```python
from build123d import *

# Parameters (mm, degrees)
SKETCH_W        = 42.5
SKETCH_H        = 70
SKETCH_R        = 11.15
SKETCH_R_2      = 1.65
SKETCH_R_3      = 2.5
PAD003_DEPTH    = 8
POCKET002_DEPTH = 4.15
SKETCH007_W     = 10
SKETCH007_H     = 70
SKETCH007_R     = 1.65
PAD004_DEPTH    = 12
SKETCH008_R     = 8.5
POCKET003_DEPTH = 12
CHAMFER004_SIZE = 3
SKETCH011_R     = 1.65
PAD005_DEPTH    = 12
CHAMFER005_SIZE = 1
SKETCH012_R     = 1.65
POCKET005_DEPTH = 8.001
SKETCH013_R     = 1.65
POCKET006_DEPTH = 20.001
SKETCH014_R     = 4
SKETCH014_R_2   = 2.5
PAD006_DEPTH    = 0.85
CHAMFER006_SIZE = 0.84
SKETCH015_R     = 1.9
POCKET007_DEPTH = 6
SKETCH016_R     = 3.15
POCKET008_DEPTH = 10.001
SKETCH017_W     = 4
SKETCH017_H     = 12.3
POCKET009_DEPTH = 12
CHAMFER007_SIZE = 1
SKETCH018_W     = 17
SKETCH018_H     = 6.956198
SKETCH018_W_2   = 15
SKETCH018_H_2   = 7.10749
SKETCH018_H_3   = 7.8
PAD007_DEPTH    = 1
CHAMFER008_SIZE = 0.99
SKETCH019_R     = 3.25
POCKET010_DEPTH = 7
SKETCH020_R     = 2
POCKET011_DEPTH = 6
CHAMFER009_SIZE = 0.4
POCKET027_DEPTH = 12
FILLET_R        = 1
SKETCH041_R     = 4.5
SKETCH041_R_2   = 2.5
PAD012_DEPTH    = 7
CHAMFER021_SIZE = 0.4


with BuildPart() as part:
    # Sketch → Pad003 (new body)
    with BuildSketch(Plane.XY):
        with Locations((21.25, 35)):
            Rectangle(SKETCH_W, SKETCH_H)
        with Locations((21.25, 48.75)):
            Circle(SKETCH_R, mode=Mode.SUBTRACT)
        with Locations((5.75, 64.25)):
            Circle(SKETCH_R_2, mode=Mode.SUBTRACT)
        with Locations((36.75, 64.25)):
            Circle(SKETCH_R_2, mode=Mode.SUBTRACT)
        with Locations((5.75, 33.25)):
            Circle(SKETCH_R_2, mode=Mode.SUBTRACT)
        with Locations((36.75, 33.25)):
            Circle(SKETCH_R_2, mode=Mode.SUBTRACT)
        with Locations((17.5, 6.74)):
            Circle(SKETCH_R_3, mode=Mode.SUBTRACT)
    extrude(amount=PAD003_DEPTH)

    # Sketch006 (on Face12 of Pad003) → Pocket002 (cut)
    with BuildSketch(Plane.XY.offset(8)):
        Polygon((42.5, 27.65), (23.35, 27.65), (20.35, 24.65), (20.35, 14.35), (23.35, 11.35), (42.5, 11.35), align=None)
    extrude(amount=-POCKET002_DEPTH, mode=Mode.SUBTRACT)

    # Sketch007 (on Face4 of Pocket002) → Pad004 (join)
    with BuildSketch(Plane.XY.offset(8)):
        with Locations((5, 35)):
            Rectangle(SKETCH007_W, SKETCH007_H)
        with Locations((5.75, 64.25)):
            Circle(SKETCH007_R, mode=Mode.SUBTRACT)
        with Locations((5.75, 33.25)):
            Circle(SKETCH007_R, mode=Mode.SUBTRACT)
    extrude(amount=PAD004_DEPTH)

    # Sketch008 (on Face4 of Pad004) → Pocket003 (cut)
    with BuildSketch(Plane.XY.offset(8)):
        with Locations((17.5, 6.74)):
            Circle(SKETCH008_R)
    extrude(amount=POCKET003_DEPTH, mode=Mode.SUBTRACT)

    # Chamfer004
    chamfer004_edges = [part.edges().sort_by_distance(p)[0] for p in [
        (42.5, 70, 4),
        (0, 70, 4),
    ]]
    chamfer(chamfer004_edges, length=CHAMFER004_SIZE)

    # Sketch011 (on Face5 of Chamfer004) → Pad005 (join)
    with BuildSketch(Plane.XY.offset(8)):
        Polygon((42.5, 67), (39.5, 70), (31.5, 70), (31.5, 59), (42.5, 59), align=None)
        with Locations((36.75, 64.25)):
            Circle(SKETCH011_R, mode=Mode.SUBTRACT)
    extrude(amount=PAD005_DEPTH)

    # Chamfer005
    chamfer005_edges = [part.edges().sort_by_distance(p)[0] for p in [
        (42.5, 59, 14),
        (31.5, 59, 14),
        (31.5, 70, 14),
        (10, 70, 14),
        (10, 0, 14),
    ]]
    chamfer(chamfer005_edges, length=CHAMFER005_SIZE)

    # Sketch012 (on Face26 of Chamfer005) → Pocket005 (cut, through all)
    with BuildSketch(Plane.XY.offset(8)):
        with Locations((32.5, 6.74)):
            Circle(SKETCH012_R)
    extrude(amount=-POCKET005_DEPTH, mode=Mode.SUBTRACT)

    # Sketch013 (on Face38 of Pocket005) → Pocket006 (cut, through all)
    with BuildSketch(Plane.XY.offset(20)):
        with Locations((5.75, 6.74)):
            Circle(SKETCH013_R)
    extrude(amount=-POCKET006_DEPTH, mode=Mode.SUBTRACT)

    # Sketch014 (on Face18 of Pocket006) → Pad006 (join)
    with BuildSketch(Plane.XY.offset(8)):
        with Locations((17.5, 6.74)):
            Circle(SKETCH014_R)
        with Locations((17.5, 6.74)):
            Circle(SKETCH014_R_2, mode=Mode.SUBTRACT)
    extrude(amount=PAD006_DEPTH)

    # Chamfer006
    chamfer006_edges = [part.edges().sort_by_distance(p)[0] for p in [
        (13.5, 6.74, 8.85),
    ]]
    chamfer(chamfer006_edges, length=CHAMFER006_SIZE)

    # Sketch015 (on Face17 of Chamfer006) → Pocket007 (cut)
    with BuildSketch(Plane.YZ.offset(42.5)):
        with Locations((6.74, 4.11193)):
            Circle(SKETCH015_R)
        with Locations((40, 4.11193)):
            Circle(SKETCH015_R)
    extrude(amount=-POCKET007_DEPTH, mode=Mode.SUBTRACT)

    # Sketch016 (on Face14 of Pocket007) → Pocket008 (cut, through all)
    with BuildSketch(Plane.YZ.offset(10)):
        with Locations((20, 14)):
            Circle(SKETCH016_R)
        with Locations((45, 14)):
            Circle(SKETCH016_R)
    extrude(amount=-POCKET008_DEPTH, mode=Mode.SUBTRACT)

    # Sketch017 (on Face36 of Pocket008) → Pocket009 (cut)
    with BuildSketch(Plane.XY.offset(20)):
        with Locations((8, 45)):
            Rectangle(SKETCH017_W, SKETCH017_H)
        with Locations((8, 20)):
            Rectangle(SKETCH017_W, SKETCH017_H)
    extrude(amount=-POCKET009_DEPTH, mode=Mode.SUBTRACT)

    # Chamfer007
    chamfer007_edges = [part.edges().sort_by_distance(p)[0] for p in [
        (10, 13.85, 14),
        (10, 26.15, 14),
        (10, 38.85, 14),
        (10, 51.15, 14),
    ]]
    chamfer(chamfer007_edges, length=CHAMFER007_SIZE)

    # Sketch018 (on Face53 of Chamfer007) → Pad007 (join)
    with BuildSketch(Plane(origin=(0, 0, 0), x_dir=(0, -1, 0), z_dir=(-1, 0, 0))):
        with Locations((-58.5, 14.421901)):
            Rectangle(SKETCH018_W, SKETCH018_H)
        with Locations((-32.5, 14.346255)):
            Rectangle(SKETCH018_W_2, SKETCH018_H_2)
        with Locations((-7.5, 14)):
            Rectangle(SKETCH018_W_2, SKETCH018_H_3)
    extrude(amount=PAD007_DEPTH)

    # Chamfer008
    chamfer008_edges = [part.edges().sort_by_distance(p)[0] for p in [
        (-1, 58.5, 10.943802),
        (-1, 32.5, 10.79251),
        (-1, 7.5, 10.1),
    ]]
    chamfer(chamfer008_edges, length=CHAMFER008_SIZE)

    # Sketch019 (on Face47 of Chamfer008) → Pocket010 (cut)
    with BuildSketch(Plane(origin=(0, 0, 0), x_dir=(1, 0, 0), z_dir=(0, 0, -1))):
        with Locations((17.5, -6.74)):
            Circle(SKETCH019_R)
    extrude(amount=-POCKET010_DEPTH, mode=Mode.SUBTRACT)

    # Sketch020 (on Face47 of Pocket010) → Pocket011 (cut)
    with BuildSketch(Plane(origin=(0, 0, 0), x_dir=(1, 0, 0), z_dir=(0, 0, -1))):
        with Locations((5.75, -6.74)):
            Circle(SKETCH020_R)
        with Locations((32.5, -6.74)):
            Circle(SKETCH020_R)
    extrude(amount=-POCKET011_DEPTH, mode=Mode.SUBTRACT)

    # Chamfer009
    chamfer009_edges = [part.edges().sort_by_distance(p)[0] for p in [
        (42.5, 33.5, 0),
        (41, 68.5, 0),
        (21.25, 0, 0),
        (21.25, 70, 0),
        (0, 33.5, 0),
        (1.5, 68.5, 0),
        (3.75, 6.74, 0),
        (14.25, 6.74, 0),
        (4.1, 33.25, 0),
        (30.5, 6.74, 0),
        (35.1, 33.25, 0),
        (4.1, 64.25, 0),
        (10.1, 48.75, 0),
        (35.1, 64.25, 0),
        (0, 41.85, 14),
        (0, 16.85, 14),
        (6, 16.85, 14),
        (6, 41.85, 14),
        (42.5, 4.84, 4.11193),
        (42.5, 38.1, 4.11193),
        (42.5, 0, 4),
    ]]
    chamfer(chamfer009_edges, length=CHAMFER009_SIZE)

    # Sketch040 (on Face78 of Chamfer009) → Pocket027 (cut)
    with BuildSketch(Plane.YZ.offset(42.5)):
        with BuildLine():
            ThreePointArc((46.75, 6), (48.75, 4), (50.75, 6))
            Line((50.75, 8), (50.75, 6))
            Line((48.75, 8), (50.75, 8))
            Line((46.75, 8), (48.75, 8))
            Line((46.75, 6), (46.75, 8))
        make_face()
    extrude(amount=-POCKET027_DEPTH, mode=Mode.SUBTRACT)

    # Fillet
    fillet_edges = [part.edges().sort_by_distance(p)[0] for p in [
        (37.359581, 46.75, 8),
        (37.359581, 50.75, 8),
    ]]
    fillet(fillet_edges, radius=FILLET_R)

    # Sketch041 (on Face62 of Fillet) → Pad012 (join)
    with BuildSketch(Plane(origin=(0, 0, 0), x_dir=(1, 0, 0), z_dir=(0, 0, -1))):
        with Locations((17.5, -6.74)):
            Circle(SKETCH041_R)
        with Locations((17.5, -6.74)):
            Circle(SKETCH041_R_2, mode=Mode.SUBTRACT)
    extrude(amount=-PAD012_DEPTH)

    # Chamfer021
    chamfer021_edges = [part.edges().sort_by_distance(p)[0] for p in [
        (15, 6.74, 0),
    ]]
    chamfer(chamfer021_edges, length=CHAMFER021_SIZE)


with BuildPart() as part_1:
    # Body placement: moved
    add(part.part.moved(Location((0, 0, 1))))


solid = part_1.part
```
Could you check a few things on this model? Use its own coordinates, in mm. A direction names the side the tool comes from. Round coordinates to 2 decimals unless told otherwise and drop trailing zeros. Loops run counter-clockwise (first coordinate to the right, second up) from the corner with the lowest first, then second, coordinate; pieces in that order, holes last. Notation, with made-up numbers: M 17.25,-6 L 65.25,-6 A17 cw 65.25,17 Z; hole C 84.5,21.25 d11. An arc over 180 degrees is marked long. Write item = value, one per line.
1. I want a section at A-A, the plane y = 33.25. Count the separate pieces of the cut face and the enclosed holes in it, and give its area (3 significant figures).
Results below:
separate_pieces = 3
enclosed_holes = 0
area = 374 mm²
2. I need wall thicknesses on probe 1 along Y at (x, z) = (5.75, 5.5); probe 2 along Y at (x, z) = (17.5, 3.5); probe 3 along Y at (x, z) = (31, 5.5). Which ranges of each line are inside material? Lowest first, please.
Results below:
probe_1 = 0 to 4.74, 8.74 to 31.6, 34.9 to 62.6, 65.9 to 70
probe_2 = 0 to 4.24, 9.24 to 38.25, 59.25 to 70
probe_3 = 0 to 5.42, 8.06 to 11.35, 27.65 to 43.34, 54.16 to 70
3. Which directions (+Z, -Z, +X, -X, +Y, -Y) give clear straight access to the entire face, cutting with the end or side of a thin tool? Please do faces 5 (the face through (24, 35, 9)), 6 (the face through (33, 11.35, 7)), 7 (the face through (10, 12, 15)).
Results below:
face_5 = +Z
face_6 = +Z, +X
face_7 = +Z, +X, +Y, -Y
4. I want a section at B-B, the plane y = 20. Write out the boundary of the cut face in (x, z).
Results below:
outline = M 0,1.4 L 0.4,1 L 42.1,1 L 42.5,1.4 L 42.5,4.85 L 20.35,4.85 L 20.35,9 L 6,9 L 6,11.45 L 5.6,11.85 L 0.4,11.85 L 0,11.45 Z; M 0,18.55 L 0.4,18.15 L 5.6,18.15 L 6,18.55 L 6,21 L 0,21 Z
5. Will these pins go through, and if not, where does the flat tip stop? P1, Ø1.1, axis at x = -0.5, z = 14.5, coming from the +Y side; P2, Ø1.9, axis at y = 40.5, z = 4.5, coming from the +X side; P3, Ø8, axis at x = 23, y = 33, coming from the +Z side.
Results below:
P1 = 67.05
P2 = 36.5
P3 = 9
6. Thinking about a two-plate mould opening in X: for faces 1 (the face through (-1, 59, 16)), 2 (the face through (35.534, 34.365, 5.147)), 3 (the face through (21.8, 12.9, 7)), 4 (the face through (15, 0, 7)), which applies, +X half, -X half, draft (parallel to the pull), parting line (faces both ways), or undercut?
Results below:
face_1 = -X half
face_2 = undercut
face_3 = +X half
face_4 = draft
